Print and shaded views of the part. All mm, measured from the part's lowest x, y and z. A direction names the side the tool comes from. Round coordinates to 2 decimals unless told otherwise and drop trailing zeros. Loops run counter-clockwise (first coordinate to the right, second up) from the corner with the lowest first, then second, coordinate; pieces in that order, holes last. Notation, with made-up numbers: (-35, 72) - (-11, 72) arc R21 cw to (-11, 79) - close; hole circle Ø5 at (17, 4). An arc over 180 degrees is marked (long way). Use one line per item in the form item = value.
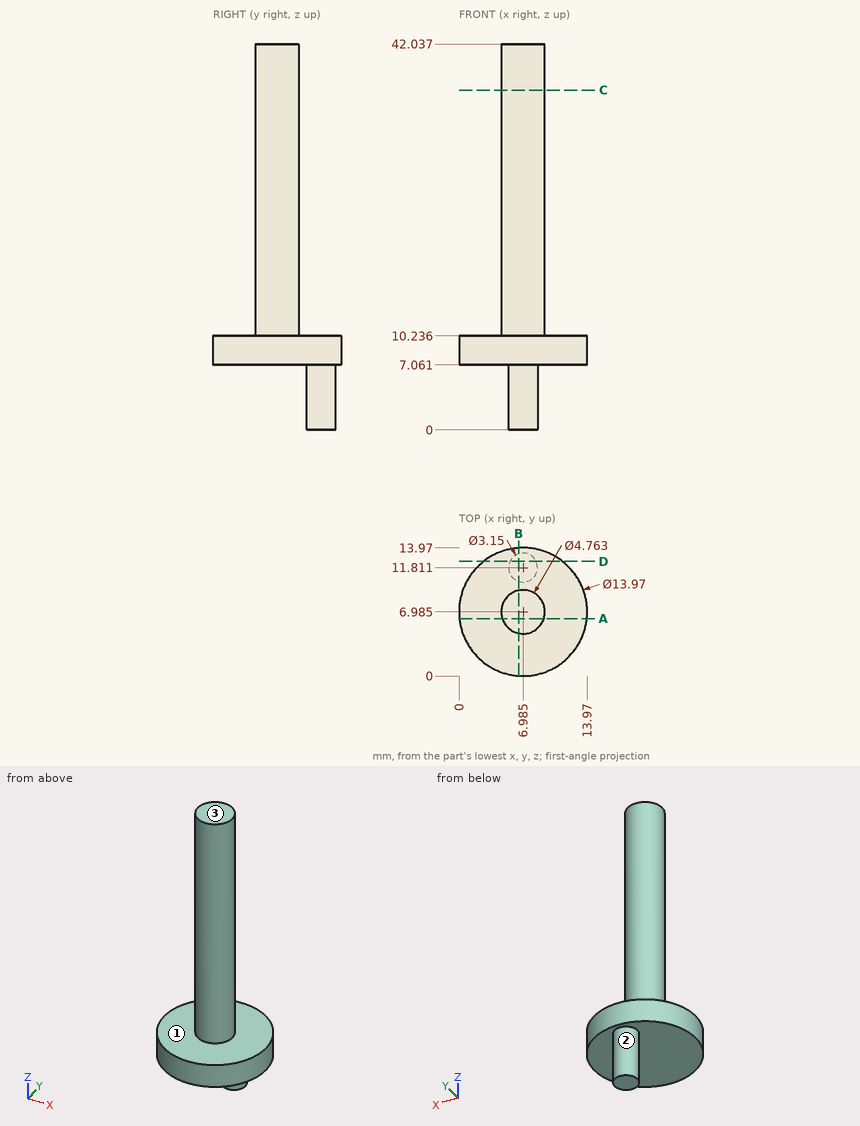
1) Drill centre lines: probe 1 along X at (y, z) = (7, 20); probe 2 along Z at (x, y) = (8, 9.75); probe 3 along Z at (x, y) = (8, 6.5). Where is each one in solid material? Low to high.
Report:
probe_1 = 4.6 to 9.37
probe_2 = 7.06 to 10.24
probe_3 = 7.06 to 42.04
2) Flat gauge pins, fed straight in: pin 1 (1.5 mm diameter, centred on x = 7, y = 10.5, fed in from +Z); pin 2 (2 mm diameter, centred on x = 7.5, y = 4.5, fed in from -Z); pin 3 (6 mm diameter, centred on x = 3, z = 19, fed in from +Y). Where does each tip first touch, or does it go through?
Report:
pin_1 = 10.24
pin_2 = 7.06
pin_3 = 9.15
3) Slice it at D-D (y = 12.5). Write the cut outline in (x, z).
Report:
outline = (2.7, 7.06) - (5.57, 7.06) - (5.57, 0) - (8.4, 0) - (8.4, 7.06) - (11.27, 7.06) - (11.27, 10.24) - (2.7, 10.24) - close
4) Slice it at A-A (y = 6.25). Write the cut outline in (x, z).
Report:
outline = (0.04, 7.06) - (13.93, 7.06) - (13.93, 10.24) - (9.25, 10.24) - (9.25, 42.04) - (4.72, 42.04) - (4.72, 10.24) - (0.04, 10.24) - close
5) Slice it at C-C (z = 37). Write the cut outline in (x, y) (1 decimal), plus the area to 3 significant figures.
Report:
outline = circle Ø4.8 at (7, 7)
area = 17.8 mm^2
6) Slice it at B-B (x = 6.5). Write the cut outline in (y, z), plus the area to 3 significant figures.
Report:
outline = (0.02, 7.06) - (10.31, 7.06) - (10.31, 0) - (13.31, 0) - (13.31, 7.06) - (13.95, 7.06) - (13.95, 10.24) - (9.32, 10.24) - (9.32, 42.04) - (4.65, 42.04) - (4.65, 10.24) - (0.02, 10.24) - close
area = 214 mm^2
7) Tool access for the marked faces 1, 2 and 3: list every direction of +Z, -Z, +X, -X, +Y, -Y with a clear straight run to the whole face (end or side of a thin tool).
Report:
face_1 = +Z
face_2 = -Z
face_3 = +Z, +X, -X, +Y, -Y
